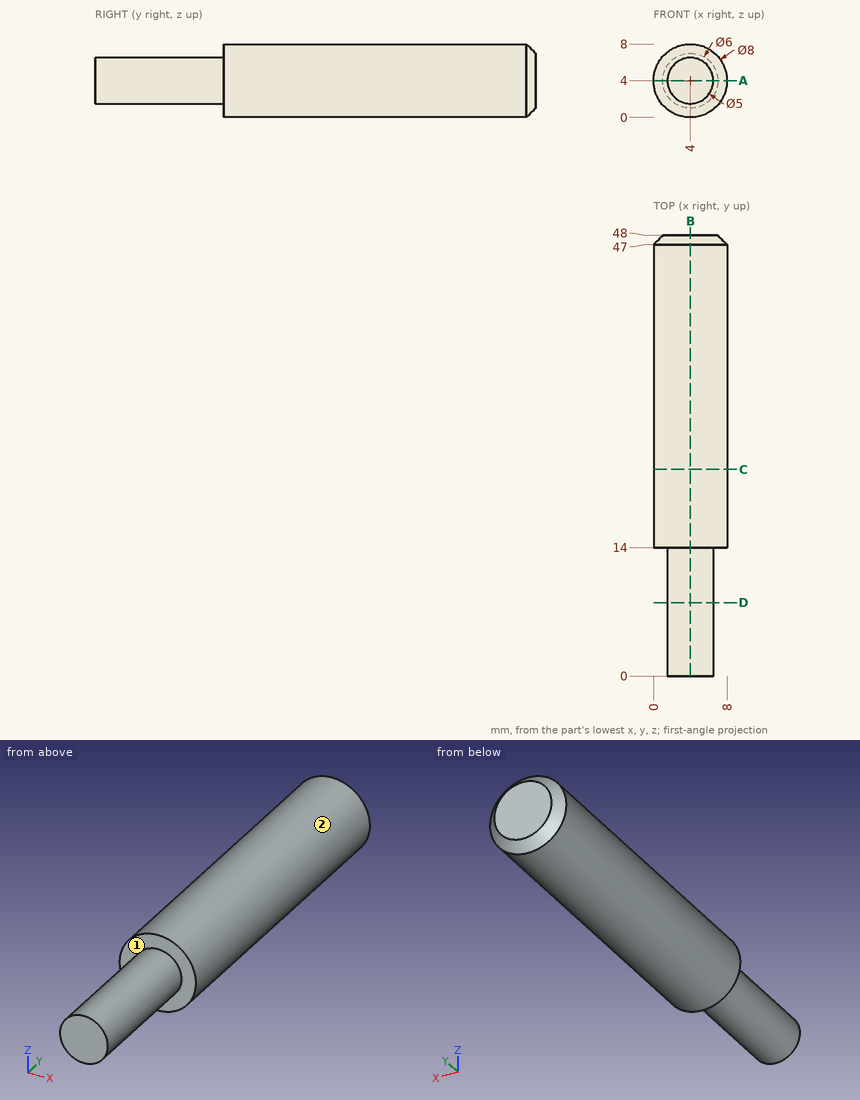
Can you work these out from the drawing? Everything is in mm from the part's minimum corner. A direction names the side the tool comes from. Coordinates: 2 decimals unless noted, no trailing zeros. Loops run counter-clockwise (first coordinate to the right, second up) from the corner with the lowest first, then second, coordinate; pieces in that order, holes last. Notation, with made-up numbers: M 38,27 L 53,27 A26 ccw 53,62 Z; hole C 66.25,21.25 d6. An arc over 180 degrees is marked long. Put each result on its own line as item: value. Start each with the question number.
(1) For the marked faces 1 and 2, which set-ups out of +Z, -Z, +X, -X, +Y, -Y let a thin tool reach every point of the face, with its end or its side?
(2) Suppose I cut it at A-A on z = 4. Please give me the cut outline in (x, y), then the cut area to 3 significant figures.
(3) I need wall thicknesses on line 1 (Y direction, x = 1.25, z = 4); line 2 (X direction, y = 28, z = 3.5); line 3 (X direction, y = 36, z = 2.5). Which ranges of each line are inside material? Lowest first, please. Write a range as from..to.
(4) Suppose I cut it at D-D on y = 8. Please give me the cut outline in (x, z).
(5) Will these pins go through, and if not, where does the flat tip stop? P1, Ø1, axis at y = 36, z = 5.5, coming from the +X side; P2, Ø1, axis at x = 6, z = 1, coming from the -Y side; P3, Ø1, axis at y = 20, z = 5, coming from the -X side.
(6) Suppose I cut it at B-B on x = 4. Please give me the cut outline in (y, z).
(7) Suppose I cut it at C-C on y = 22.5. Please give me the cut outline in (x, z).
Solutions:
1. face 1: -Y
1. face 2: +Y, -Y
2. outline: M 0,14 L 1.5,14 L 1.5,0 L 6.5,0 L 6.5,14 L 8,14 L 8,47 L 7,48 L 1,48 L 0,47 Z
2. area: 341 mm2
3. line 1: y = 14..48
3. line 2: x = 0.03..7.97
3. line 3: x = 0.29..7.71
4. outline: C 4,4 d5
5. P1: stops at x = 7.87
5. P2: stops at y = 14
5. P3: stops at x = 0.03
6. outline: M 0,1.5 L 14,1.5 L 14,0 L 47,0 L 48,1 L 48,7 L 47,8 L 14,8 L 14,6.5 L 0,6.5 Z
7. outline: C 4,4 d8
